For this review, use the dimensioned drawing (mm, ordinates from the lowest corner) and the shaded views. A direction names the side the tool comes from. Coordinates: 2 decimals unless noted, no trailing zeros. Loops run counter-clockwise (first coordinate to the right, second up) from the corner with the lowest first, then second, coordinate; pieces in that order, holes last. Notation, with made-up numbers: (38.25, -36) - (71.25, -36) arc R8 cw to (71.25, -23) - close; hole circle Ø2 at (27, 81.5). An arc over 180 degrees is marked (long way). Answer in a Markdown table with one row per item. Add a question column.
(1) We need section A-A, the plane z = 1. Write out the cut boundary in (x, y).
(2) We need section B-B, the plane y = 4. Write out the cut boundary in (x, z).
(3) We need section C-C, the plane x = 9.75. Write out the cut boundary in (y, z).
(4) The part is to be moulded in two halves that separate along X. For the marked faces 4, 5 and 6, say which applies: released by +X, released by -X, zero draft, split by the parting line, or undercut.
(5) Clearance check with flat-ended pins moving along their axes: pin 1 (0.9 mm diameter, centred on x = 3, y = 13, fed in from +Z); pin 2 (2 mm diameter, centred on x = 9.5, y = 4.5, fed in from +Z). State where each tip first meets the part, or that it passes through.
(6) We need section D-D, the plane x = 3.5. Write out the cut boundary in (y, z).
(7) To check wall thickness, follow L1, parallel to Y at x = 23.5, z = 9.25; L2, parallel to X at y = 12.7, z = 8.1; L3, parallel to Y at x = 4.75, z = 9. State the ranges of each line that lie inside material, in increasing order. Write a range as [from, to].
(8) For the marked faces 1, 2 and 3, list the 3-axis set-ups (+Z, -Z, +X, -X, +Y, -Y) from which the entire face can be reached by the end or side of a thin tool; tool diameter is ignored.
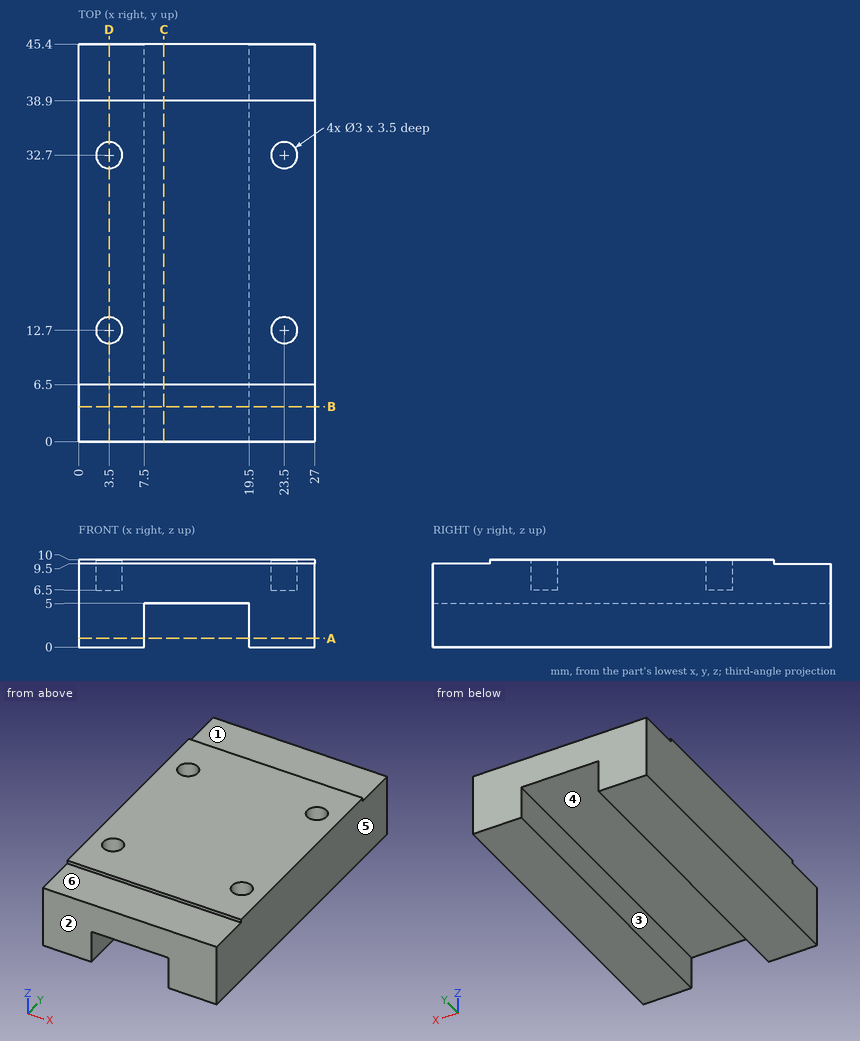
Responses:
| question | item | result |
|---|---|---|
| 1 | outline | (0, 0) - (7.5, 0) - (7.5, 45.4) - (0, 45.4) - close; (19.5, 0) - (27, 0) - (27, 45.4) - (19.5, 45.4) - close |
| 2 | outline | (0, 0) - (7.5, 0) - (7.5, 5) - (19.5, 5) - (19.5, 0) - (27, 0) - (27, 9.5) - (0, 9.5) - close |
| 3 | outline | (0, 5) - (45.4, 5) - (45.4, 9.5) - (38.9, 9.5) - (38.9, 10) - (6.5, 10) - (6.5, 9.5) - (0, 9.5) - close |
| 4 | face 4 | undercut |
| 4 | face 5 | released by +X |
| 4 | face 6 | zero draft |
| 5 | pin 1 | stops at z = 6.5 |
| 5 | pin 2 | stops at z = 9.5 |
| 6 | outline | (0, 0) - (45.4, 0) - (45.4, 9.5) - (38.9, 9.5) - (38.9, 10) - (34.2, 10) - (34.2, 6.5) - (31.2, 6.5) - (31.2, 10) - (14.2, 10) - (14.2, 6.5) - (11.2, 6.5) - (11.2, 10) - (6.5, 10) - (6.5, 9.5) - (0, 9.5) - close |
| 7 | L1 | y = [0, 11.2], [14.2, 31.2], [34.2, 45.4] |
| 7 | L2 | x = [0, 2], [5, 22], [25, 27] |
| 7 | L3 | y = [0, 11.87], [13.53, 31.87], [33.53, 45.4] |
| 8 | face 1 | +Z, +X, -X, +Y |
| 8 | face 2 | +Z, -Z, +X, -X, -Y |
| 8 | face 3 | -Z, +Y, -Y |
